Design review of the part built by this model. Coordinates are the model's own, in mm. A direction names the side the tool comes from. Coordinates: 2 decimals unless noted, no trailing zeros. Write each loop counter-clockwise with the first axis right and the second up, starting at its lowest first coordinate (ties: lowest second). Pieces come first, ordered by that corner, then holes.
Q1. The part is to be moulded in two halves that separate along Y. For faces 1 (the flat face through (0, -23, 3.2)), 2 (the flat face through (0, -20.066, -1)), 3 (the flat face through (-3.998, -23, 2)), 4 (the flat face through (1, -23.741, 5)), say which applies: released by +Y, released by -Y, zero draft, split by the parting line, or undercut.
Q2. Take a section at A-A, the plane z = 4.5. Write out the cut boundary in (x, y), plus the area to 3 significant figures.
Q3. Take a section at D-D, the plane x = -2.5. Write out the cut boundary in (y, z).
Q4. Take a section at C-C, the plane x = 0.5. Write out the cut boundary in (y, z).
Q5. For L1, parallel to Z at x = 0, y = -26; L2, parallel to X at y = -24.5, z = 5.75; L3, parallel to Y at x = 0.5, z = 6.75, list the stretches that pass through material, from the lowest coordinate up.
Q6. For pin 1 Ø1.1 at (x, z) = (-1.5, 6.5) entering from +Y; pin 2 Ø1.5 at (y, z) = (-24.5, 4.5) entering from +X; pin 3 Ø1.5 at (y, z) = (-24, 5.5) entering from -X, all flat-tipped, find the tip position at first contact; note any pin that passes through.
Q7. For faces 5 (the flat face through (4.002, -23, 2)), 6 (the flat face through (3.002, -23, -1)), 7 (the flat face through (-2.998, -23, -1)), 8 (the flat face through (0.677, -24, 5)), list the 3-axis set-ups (+Z, -Z, +X, -X, +Y, -Y) from which the entire face can be reached by the end or side of a thin tool; tool diameter is ignored.
Q8. Take a section at B-B, the plane y = -24.75. Write out the cut boundary in (x, z), plus the area to 3 significant figures.
from build123d import *

# Parameters (mm, degrees)
BOSS_EXTRUDE1_DEPTH = 7.5
SKETCH7_W           = 8
SKETCH7_H           = 8
BOSS_EXTRUDE2_DEPTH = 3.2
SKETCH8_W           = 6
SKETCH8_H           = 6
BOSS_EXTRUDE3_DEPTH = 1.3


with BuildPart() as part:
    # Sketch6 → Boss-Extrude1 (new body)
    with BuildSketch(Plane(origin=(0, 4.132474232, 0), x_dir=(-1, 0, 0), z_dir=(0, 0, 1))):
        with BuildLine():
            ThreePointArc((-2.772388639, 27.198186003), (-1.961074426, 25.239500222), (-0.002388647, 24.428186003))
            ThreePointArc((-0.002388647, 24.428186003), (1.956297142, 25.239500216), (2.767611361, 27.198186003))
            ThreePointArc((2.767611361, 27.198186003), (1.956297145, 29.156871787), (-0.002388639, 29.968186003))
            ThreePointArc((-0.002388639, 29.968186003), (-1.961074423, 29.156871787), (-2.772388639, 27.198186003))
        make_face()
        Polygon((2.047611361, 27.873186003), (2.047611361, 26.523186003), (0.672611361, 26.523186003), (0.672611361, 25.148186003), (-0.677388639, 25.148186003), (-0.677388639, 26.523186003), (-2.052388639, 26.523186003), (-2.052388639, 27.873186003), (-0.677388639, 27.873186003), (-0.677388639, 29.248186003), (0.672611361, 29.248186003), (0.672611361, 27.873186003), align=None, mode=Mode.SUBTRACT)
    extrude(amount=BOSS_EXTRUDE1_DEPTH)

    # Sketch7 → Boss-Extrude2 (add)
    with BuildSketch(Plane(origin=(0, 0, 0), x_dir=(-1, 0, 0), z_dir=(0, 0, 1))):
        with Locations((-0.002388639, 23.065711771)):
            Rectangle(SKETCH7_W, SKETCH7_H)
    extrude(amount=BOSS_EXTRUDE2_DEPTH)

    # Sketch8 → Boss-Extrude3 (add)
    with BuildSketch(Plane(origin=(0, 0, 0), x_dir=(-1, 0, 0), z_dir=(0, 0, -1))):
        with Locations((-0.002388639, -23.065711771)):
            Rectangle(SKETCH8_W, SKETCH8_H)
    extrude(amount=BOSS_EXTRUDE3_DEPTH)


solid = part.part
Responses:
1. face 1: undercut
1. face 2: released by +Y
1. face 3: zero draft
1. face 4: undercut
2. outline: circle Ø5.54 at (0, -23.07); hole (-2.05, -23.74) - (-0.67, -23.74) - (-0.67, -25.12) - (0.68, -25.12) - (0.68, -23.74) - (2.05, -23.74) - (2.05, -22.39) - (0.68, -22.39) - (0.68, -21.02) - (-0.67, -21.02) - (-0.67, -22.39) - (-2.05, -22.39) - close
2. area: 14.9 mm2
3. outline: (-27.07, 0) - (-26.07, 0) - (-26.07, -1.3) - (-20.07, -1.3) - (-20.07, 0) - (-19.07, 0) - (-19.07, 3.2) - (-21.88, 3.2) - (-21.88, 7.5) - (-24.25, 7.5) - (-24.25, 3.2) - (-27.07, 3.2) - close
4. outline: (-27.07, 0) - (-26.07, 0) - (-26.07, -1.3) - (-20.07, -1.3) - (-20.07, 0) - (-19.07, 0) - (-19.07, 3.2) - (-20.34, 3.2) - (-20.34, 7.5) - (-21.02, 7.5) - (-21.02, 3.2) - (-25.12, 3.2) - (-25.12, 7.5) - (-25.79, 7.5) - (-25.79, 3.2) - (-27.07, 3.2) - close
5. L1: z = -1.3 to 3.2
5. L2: x = -2.37 to -0.67, 0.68 to 2.37
5. L3: y = -25.79 to -25.12, -21.02 to -20.34
6. pin 1: stops at y = -20.46
6. pin 2: stops at x = 2.69
6. pin 3: stops at x = -2.76
7. face 5: +Z, -Z, +X, +Y, -Y
7. face 6: -Z, +X, +Y, -Y
7. face 7: -Z, -X, +Y, -Y
7. face 8: +Z
8. outline: (-4, 0) - (-3, 0) - (-3, -1.3) - (3, -1.3) - (3, 0) - (4, 0) - (4, 3.2) - (2.2, 3.2) - (2.2, 7.5) - (0.68, 7.5) - (0.68, 3.2) - (-0.67, 3.2) - (-0.67, 7.5) - (-2.2, 7.5) - (-2.2, 3.2) - (-4, 3.2) - close
8. area: 46.5 mm2
